```python
from build123d import *

# Parameters (mm, degrees)
F0_W = 42.2452799976
F0_H = 53.2546564937
F2_T = -2.54
F3_R = 1.26999
F4_R = 1.27


# Not quite as in the source:
# - a fillet or chamfer is up to 0.001 mm smaller than in the source, because OpenCascade refuses the exact size


with BuildPart() as f1:
    # F0 (on Front) → F1 (revolve)
    with BuildSketch(Plane.XZ):
        with Locations((-21.1226399988, 1.152144745)):
            Rectangle(F0_W, F0_H)
    revolve(axis=Axis((0, 0, 1.152144745), (0, 0, 1)))

    # F2
    f2_openings = [f1.faces().sort_by_distance(p)[0] for p in [
        (0, 0, 27.779473),
    ]]
    offset(amount=F2_T, openings=f2_openings)

    # F3 (radius 1.27 in the source; OpenCascade refuses exactly that, so slightly less here)
    f3_edges = [f1.edges().sort_by_distance(p)[0] for p in [
        (39.70528, 0, 27.779473),
        (42.24528, 0, 27.779473),
    ]]
    fillet(f3_edges, radius=F3_R)

    # F4
    f4_edges = [f1.edges().sort_by_distance(p)[0] for p in [
        (39.70528, 0, -22.935184),
        (42.24528, 0, -25.475184),
    ]]
    fillet(f4_edges, radius=F4_R)


solid = f1.part
```
The model under review builds one solid part; all positions refer to its coordinate system, in mm. Round coordinates to 2 decimals unless told otherwise and drop trailing zeros. Order: outer loops, then holes, each group sorted by start corner. A loop starts at its lowest first (then second) coordinate and runs counter-clockwise, first axis right, second up.
Item 1: For pin 1 (8 mm diameter, centred on x = 20.5, z = 15.5, fed in from +Y); pin 2 (1.5 mm diameter, centred on x = 19.5, y = 2.5, fed in from +Z); pin 3 (4 mm diameter, centred on x = 19.5, z = -4.5, fed in from +Y), all flat-tipped, find the tip position at first contact; note any pin that passes through.
Working result:
pin 1: stops at y = 38.89
pin 2: stops at z = -22.94
pin 3: stops at y = 38.45
Item 2: Draft analysis for pull direction X (two halves, no side actions). For faces 1 (the cylindrical face through (-36.678, 15.207, 2.759)), 2 (the flat face through (1, -1, -25.475)), 3 (the cylindrical face through (9.16, 41.24, 1.51)), state which applies: released by +X, released by -X, zero draft, split by the parting line, or undercut.
Working result:
face 1: undercut
face 2: zero draft
face 3: split by the parting line
Item 3: To check wall thickness, follow probe 1 along Y at (x, z) = (0, 13); probe 2 along Z at (x, y) = (11, 29.5). State the ranges of each line that lie inside material, in increasing order.
Working result:
probe 1: y = -42.25 to -39.71, 39.71 to 42.25
probe 2: z = -25.48 to -22.94
Item 4: Add section C-C, the plane z = -19.5. State the section outline as (x, y) points, and give its area (3 significant figures).
Working result:
outline: circle Ø84.49 at (0, 0); hole circle Ø79.41 at (0, 0)
area: 654 mm2
